The model under review builds one solid part; all positions refer to its coordinate system, in mm. Face numbers are marked on the shaded views. A direction names the side the tool comes from. Give positions to 0.01 mm unless a question says otherwise; leave off trailing zeros. Write each loop counter-clockwise with the first axis right and the second up, starting at its lowest first coordinate (ties: lowest second). Pieces come first, ordered by that corner, then holes. Notation, with made-up numbers: (52, 7) - (68, 7) arc R18 cw to (68, 15) - close; hole circle Ø3 at (-34, 40). An arc over 180 degrees is marked (long way). Write item = value, one per line.
```python
from build123d import *

# Parameters (mm, degrees)
CUT_EXTRUDE1_DEPTH      = 42.656
CUT_EXTRUDE1_DEPTH_BACK = 42.656


with BuildPart() as part:
    # Sketch1 → CHAMBER GEOMETRY (revolve)
    with BuildSketch(Plane.XY):
        with BuildLine():
            Line((0, 0), (-38.1, 0))
            Line((-38.1, 0), (-38.1, -157.332041631))
            Line((-38.1, -157.332041631), (-19.331058169, -208.113159893))
            ThreePointArc((-19.331058169, -208.113159893), (-18.081947937, -212.694672543), (-17.653, -217.424))
            ThreePointArc((-17.653, -217.424), (-17.710909205, -218.322313303), (-17.888255676, -219.204848569))
            Line((-17.888255676, -219.204848569), (-41.656, -307.594))
            Line((-41.656, -307.594), (0, -307.594))
            Line((0, -307.594), (0, 0))
        make_face()
    revolve(axis=Axis((0, 0, 0), (0, -1, 0)))

    # Sketch3 → CF REVOLVE (revolve)
    with BuildSketch(Plane.XY):
        with BuildLine():
            ThreePointArc((19.052545295, -218.891772388), (18.923521318, -218.163557003), (18.923, -217.424))
            ThreePointArc((18.923, -217.424), (19.548451138, -212.730087586), (20.601058169, -208.113159893))
            Line((20.601058169, -208.113159893), (19.331058169, -208.113159893))
            ThreePointArc((19.331058169, -208.113159893), (18.081947937, -212.694672543), (17.653, -217.424))
            ThreePointArc((17.653, -217.424), (17.710909205, -218.322313303), (17.888255676, -219.204848569))
            Line((17.888255676, -219.204848569), (19.254262016, -224.284848569))
            Line((19.254262016, -224.284848569), (20.418551634, -223.971772388))
            Line((20.418551634, -223.971772388), (19.052545295, -218.891772388))
        make_face()
        Polygon((24.927703857, -196.634205845), (23.736466151, -196.193918747), (19.331058169, -208.113159893), (20.601058169, -208.113159893), align=None)
        Polygon((39.453969902, -157.332041631), (38.1, -157.332041631), (23.736466151, -196.193918747), (24.927703857, -196.634205845), align=None)
        Polygon((39.453969902, -132.003733221), (37.984578859, -132.003733221), (38.1, -157.332041631), (39.453969902, -157.332041631), align=None)
    revolve(axis=Axis((0, -217.424, 0), (0, 1, 0)))

    # Sketch4 → RTV/EPOXY (revolve)
    with BuildSketch(Plane.XY):
        Polygon((18.923521318, -218.163557003), (18.923521318, -213.083557003), (20.955521318, -213.083557003), (20.955521318, -221.211557003), (18.923521318, -221.211557003), align=None)
    revolve(axis=Axis((0, -217.424, 0), (0, -1, 0)))

    # Sketch6 → Cut-Extrude1 (cut, two sides)
    with BuildSketch(Plane.XY) as cut_extrude1_sk:
        Polygon((41.656, -307.594), (21.870533279, -234.014421294), (-21.870533279, -234.014421294), (-41.656, -307.594), align=None)
    extrude(amount=CUT_EXTRUDE1_DEPTH, mode=Mode.SUBTRACT)
    extrude(cut_extrude1_sk.sketch, amount=-CUT_EXTRUDE1_DEPTH_BACK, mode=Mode.SUBTRACT)

    # Sketch7 → DASHED RTV/EPOXY (revolve)
    with BuildSketch(Plane(origin=(0, 0, 0), x_dir=(0, 0, -1), z_dir=(1, 0, 0))):
        Polygon((-21.870533279, -234.014421294), (-42.359549747, -310.214421294), (0, -310.214421294), (0, -234.014421294), align=None)
    revolve(axis=Axis((0, -310.214421294, 0), (0, 1, 0)))

    # Sketch10 → DASHED RTV/EPOXY OVERHANG (revolve)
    with BuildSketch(Plane.XY):
        Polygon((21.870533279, -204.745135906), (34.75998975, -170.032041631), (34.75998975, -250.042041631), (26.180115655, -250.042041631), (21.870533279, -234.014421294), align=None)
    revolve(axis=Axis((0, -221.211557003, 0), (0, 1, 0)))

    # Sketch11 → BLUE TUBE (revolve)
    with BuildSketch(Plane.XY):
        Polygon((34.75998975, -253.947859685), (27.23033049, -253.947859685), (25.282654818, -253.947859685), (25.282654818, -250.042041631), (27.23033049, -250.042041631), (34.75998975, -250.042041631), (38.1, -250.042041631), (38.1, -132.003733221), (38.1, 0), (38.1, 8.89), (57.15, 8.89), (57.15, 0), (46.584796967, 0), (46.584796967, -253.947859685), align=None)
    revolve(axis=Axis((0, 0, 0), (0, -1, 0)))


solid = part.part
```
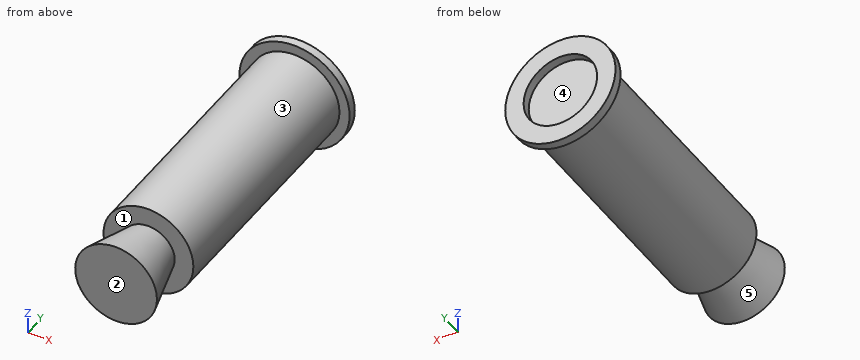
1. Take a section at A-A on x = -26. Count the separate pieces of the cut face and the enclosed holes in it, and give its area (3 significant figures).
Findings below:
separate_pieces = 1
enclosed_holes = 2
area = 21,800 mm²
2. Draft analysis for pull direction Y (two halves, no side actions). For the marked faces 3, 4 and 5, state which applies: +Y half, -Y half, draft (parallel to the pull), parting line (faces both ways), or undercut.
Findings below:
face_3 = draft
face_4 = +Y half
face_5 = undercut
3. For line 1 (Z direction, x = 0, y = -217); line 2 (Z direction, x = 0, y = 6); line 3 (X direction, y = -194.5, z = -10), list the stretches that pass through material, from the lowest coordinate up. Write a range as from..to.
Findings below:
line_1 = -46.58..-38.1, -34.76..-21.87, -20.96..20.96, 21.87..34.76, 38.1..46.58
line_2 = -57.15..-38.1, 38.1..57.15
line_3 = -45.5..-36.76, -33.29..33.29, 36.76..45.5
4. Insertion check: P1, Ø5, axis at y = -245, z = 33.5, coming from the -X side; P2, Ø5, axis at x = 2, y = -78, coming from the +Z side; P3, Ø23, axis at x = -11, z = 14, coming from the +Y side. Each pin has a flat end and moves straight along its axis. Give the tip position at first contact, or say it passes through.
Findings below:
P1 = -34.77
P2 = 46.58
P3 = 0
5. Machinability: for the marked faces 1 and 2, which of the approach directions +Z, -Z, +X, -X, +Y, -Y give a long, thin tool a straight path to every point of the face, cutting with its end or side? Answer none if there is none.
Findings below:
face_1 = none
face_2 = +Z, -Z, +X, -X, -Y
6. Take a section at C-C on y = -28. Give the boundary of the cut face in (x, z), and give its area (3 significant figures).
Findings below:
outline = circle Ø93.17 at (0, 0)
area = 6,820 mm²
